Build history of the part. All positions in model axes, mm. Face numbers are marked on the shaded views. A direction names the side the tool comes from. Give positions to 0.01 mm unless a question says otherwise; leave off trailing zeros. Loops run counter-clockwise (first coordinate to the right, second up) from the corner with the lowest first, then second, coordinate; pieces in that order, holes last. Notation, with made-up numbers: (-11, 47.25) - (22, 47.25) arc R27 cw to (22, 63.25) - close; hole circle Ø3 at (72, 73). An arc over 180 degrees is marked (long way). Return JSON: item names as keys, results as strings. Group by question number.
1) Slice it at A-A (z = -26.5). List the corners of the cut face in (x, y), and give its area (3 significant figures).
2) Mould opens along Y. For the marked faces 1, 2 and 3 say: released by +Y, released by -Y, zero draft, split by the parting line, or undercut.
3) Slice it at C-C (y = 14). List the corners of the cut face in (x, z).
4) 3-axis set-ups, long thin cutter, end or side, ignore diameter. For the marked faces 4, 5, 6, 7 and 8: which of +Z, -Z, +X, -X, +Y, -Y reach the whole face in a straight line?
5) Slice it at B-B (x = 26.5). List the corners of the cut face in (y, z), and give its area (3 significant figures).
6) Slice it at D-D (z = -11). List the corners of the cut face in (x, y).
7) Drill centre lines: probe 1 along Z at (x, y) = (47.5, 4); probe 2 along X at (y, z) = (10.5, -23); probe 3 along Y at (x, z) = (44, -5). Where is each one in solid material? Low to high. Write a range as from..to.
8) Drop flat-ended pins along their axis: pin 1 (1 mm diameter, centred on x = 31, y = 4, fed in from +Z); pin 2 (5.5 mm diameter, centred on x = 10.35, y = 10.35, fed in from -Z); pin 3 (1.5 mm diameter, centred on x = 20.5, y = -16, fed in from -Z); pin 4 (5.5 mm diameter, centred on x = 9, y = 14, fed in from -Z). Give the stop position or say it passes through.
```python
from build123d import *

# Parameters (mm, degrees)
BOSS_EXTRUDE1_DEPTH  = 20.701
SKETCH2_R            = 1
CUT_EXTRUDE1_DEPTH   = 93.545558787
SKETCH3_R            = 1
CUT_EXTRUDE2_DEPTH   = 12.7
SKETCH4_R            = 1
BOSS_EXTRUDE3_DEPTH  = 5.08
SKETCH5_W            = 5.08
SKETCH5_H            = 5.08
BOSS_EXTRUDE4_DEPTH  = 5.08
SKETCH6_W            = 5.08
SKETCH6_H            = 5.08
BOSS_EXTRUDE5_DEPTH  = 5.08
SKETCH7_W            = 2.54
SKETCH7_H            = 15
CUT_EXTRUDE3_DEPTH   = 108.238791728
SKETCH8_W            = 25.4
SKETCH8_H            = 32.87751569
CUT_EXTRUDE4_DEPTH   = 99.137252123
BOSS_EXTRUDE6_DEPTH  = 5.08
BOSS_EXTRUDE9_START  = -5.08
SKETCH12_R           = 1
BOSS_EXTRUDE9_DEPTH  = 5.08
SKETCH13_R           = 1
BOSS_EXTRUDE10_DEPTH = 24.4
CUT_EXTRUDE5_DEPTH   = 30
SKETCH11_R           = 4.5
CUT_EXTRUDE6_DEPTH   = 40
SKETCH16_R           = 3.175
SKETCH16_R_2         = 4.7625
SKETCH16_R_3         = 2.5
CUT_EXTRUDE7_DEPTH   = 40


with BuildPart() as part:
    # Sketch1 → Boss-Extrude1 (new body)
    with BuildSketch(Plane(origin=(0, 0, 0), x_dir=(1, 0, 0), z_dir=(0, 1, 0))):
        Polygon((86.5505, 0), (86.5505, 25.4), (81.4705, 25.4), (81.4705, 10.16), (76.3905, 5.08), (81.4705, 5.08), (81.4705, 0), align=None)
        Polygon((20.701, 10.16), (20.701, 25.4), (0, 25.4), (0, 0), (81.4705, 0), (81.4705, 5.08), (76.3905, 5.08), (25.781, 5.08), (20.701, 5.08), align=None)
        Polygon((20.701, 10.16), (25.781, 5.08), (20.701, 5.08), align=None)
    extrude(amount=BOSS_EXTRUDE1_DEPTH)

    # Sketch2 → Cut-Extrude1 (cut, through all)
    with BuildSketch(Plane(origin=(0, 0, -25.4), x_dir=(-1, 0, 0), z_dir=(0, 0, -1))):
        with Locations((-10.3505, 10.3505)):
            Circle(SKETCH2_R)
    extrude(amount=-CUT_EXTRUDE1_DEPTH, mode=Mode.SUBTRACT)

    # Sketch3 → Cut-Extrude2 (cut)
    with BuildSketch(Plane.XY):
        with Locations((50.970999912, 10.3505)):
            Circle(SKETCH3_R)
    extrude(amount=-CUT_EXTRUDE2_DEPTH, mode=Mode.SUBTRACT)

    # Sketch4 → Boss-Extrude3 (add)
    with BuildSketch(Plane.XY):
        with BuildLine():
            Line((40.280941282, 0), (27.580941282, 0))
            Line((27.580941282, 0), (25.4, 0))
            Line((25.4, 0), (0, 0))
            Line((0, 0), (16.608872552, -28.493600659))
            ThreePointArc((16.608872552, -28.493600659), (30.893397103, -34.358409309), (40.280941282, -22.098))
            Line((40.280941282, -22.098), (40.280941282, 0))
        make_face()
        with Locations((20.138741282, -22.098)):
            Circle(SKETCH4_R, mode=Mode.SUBTRACT)
        with BuildLine():
            ThreePointArc((26.580941282, -22.098), (26.873834501, -21.390893219), (27.580941282, -21.098))
            ThreePointArc((27.580941282, -21.098), (28.288048063, -21.390893219), (28.580941282, -22.098))
            ThreePointArc((28.580941282, -22.098), (27.580941282, -23.098), (26.580941282, -22.098))
        make_face(mode=Mode.SUBTRACT)
        with BuildLine():
            ThreePointArc((36.023141282, -22.098), (35.023141282, -23.098), (34.023141282, -22.098))
            ThreePointArc((34.023141282, -22.098), (35.023141282, -21.098), (36.023141282, -22.098))
        make_face(mode=Mode.SUBTRACT)
    extrude(amount=-BOSS_EXTRUDE3_DEPTH)

    # Sketch5 → Boss-Extrude4 (add)
    with BuildSketch(Plane(origin=(0, 0, -25.4), x_dir=(-1, 0, 0), z_dir=(0, 0, -1))):
        with Locations((-2.54, 2.54)):
            Rectangle(SKETCH5_W, SKETCH5_H)
        with Locations((-2.54, 18.161)):
            Rectangle(SKETCH5_W, SKETCH5_H)
        with Locations((-18.161, 18.161)):
            Rectangle(SKETCH5_W, SKETCH5_H)
        with Locations((-18.161, 2.54)):
            Rectangle(SKETCH5_W, SKETCH5_H)
    extrude(amount=BOSS_EXTRUDE4_DEPTH)

    # Sketch6 → Boss-Extrude5 (add)
    with BuildSketch(Plane(origin=(0, 0, -25.4), x_dir=(-1, 0, 0), z_dir=(0, 0, -1))):
        with Locations((-84.0105, 18.161)):
            Rectangle(SKETCH6_W, SKETCH6_H)
        with Locations((-84.0105, 2.54)):
            Rectangle(SKETCH6_W, SKETCH6_H)
    extrude(amount=BOSS_EXTRUDE5_DEPTH)

    # Sketch7 → Cut-Extrude3 (cut, through all)
    with BuildSketch(Plane(origin=(0, 20.701, 0), x_dir=(1, 0, 0), z_dir=(0, 1, 0))):
        with Locations((82.7405, 22.98)):
            Rectangle(SKETCH7_W, SKETCH7_H)
        with Locations((19.431, 22.98)):
            Rectangle(SKETCH7_W, SKETCH7_H)
    extrude(amount=-CUT_EXTRUDE3_DEPTH, mode=Mode.SUBTRACT)

    # Sketch8 → Cut-Extrude4 (cut, through all)
    with BuildSketch(Plane(origin=(0, 0, 0), x_dir=(-1, 0, 0), z_dir=(0, -1, 0))):
        with Locations((-73.8505, 16.438757845)):
            Rectangle(SKETCH8_W, SKETCH8_H)
    extrude(amount=-CUT_EXTRUDE4_DEPTH, mode=Mode.SUBTRACT)

    # Sketch9 → Boss-Extrude6 (add)
    with BuildSketch(Plane.XY):
        with BuildLine():
            Line((8.304436276, -28.493600659), (16.608872552, -28.493600659))
            Line((16.608872552, -28.493600659), (0, 0))
            Line((0, 0), (0, -14.24680033))
            Line((0, -14.24680033), (3.648627535, -20.506258075))
            ThreePointArc((3.648627535, -20.506258075), (4.650419602, -20.503139192), (5.152218138, -21.370200495))
            ThreePointArc((5.152218138, -21.370200495), (5.01927944, -21.868401958), (4.655808741, -22.234142914))
            Line((4.655808741, -22.234142914), (8.304436276, -28.493600659))
        make_face()
        with BuildLine():
            Line((0, -28.493600659), (8.304436276, -28.493600659))
            Line((8.304436276, -28.493600659), (4.655808741, -22.234142914))
            ThreePointArc((4.655808741, -22.234142914), (3.288275718, -21.873791098), (3.648627535, -20.506258075))
            Line((3.648627535, -20.506258075), (0, -14.24680033))
            Line((0, -14.24680033), (0, -28.493600659))
        make_face()
    extrude(amount=-BOSS_EXTRUDE6_DEPTH)

    # Sketch12 → Boss-Extrude9 (add)
    with BuildSketch(Plane(origin=(0, 0, -5.08), x_dir=(-1, 0, 0), z_dir=(0, 0, -1)).offset(BOSS_EXTRUDE9_START)):
        with Locations((-4.152218138, -21.370200495)):
            Circle(SKETCH12_R)
        with Locations((-20.138741282, -22.098)):
            Circle(SKETCH12_R)
        with Locations((-27.580941282, -22.098)):
            Circle(SKETCH12_R)
        with Locations((-35.023141282, -22.098)):
            Circle(SKETCH12_R)
        with Locations((-50.970999912, 10.3505)):
            Circle(SKETCH12_R)
    extrude(amount=BOSS_EXTRUDE9_DEPTH)

    # Sketch13 → Boss-Extrude10 (add)
    with BuildSketch(Plane(origin=(0, 0, -25.4), x_dir=(-1, 0, 0), z_dir=(0, 0, -1))):
        with Locations((-10.3505, 10.3505)):
            Circle(SKETCH13_R)
    extrude(amount=-BOSS_EXTRUDE10_DEPTH)

    # Sketch15 → Cut-Extrude5 (cut)
    with BuildSketch(Plane(origin=(0, 20.701, 0), x_dir=(1, 0, 0), z_dir=(0, 1, 0))):
        Polygon((18.161, 15.48), (18.161, 12.717664049), (20.701, 10.16), (20.701, 15.48), align=None)
    extrude(amount=-CUT_EXTRUDE5_DEPTH, mode=Mode.SUBTRACT)

    # Sketch11 → Cut-Extrude6 (cut)
    with BuildSketch(Plane.XY):
        with Locations((10.3505, 10.3505)):
            Circle(SKETCH11_R)
    extrude(amount=-CUT_EXTRUDE6_DEPTH, mode=Mode.SUBTRACT)

    # Sketch16 → Cut-Extrude7 (cut)
    with BuildSketch(Plane.XY):
        with Locations((27.580941282, -22.098)):
            Circle(SKETCH16_R)
        with Locations((50.970999912, 10.3505)):
            Circle(SKETCH16_R_2)
        with Locations((4.152218138, -21.370200495)):
            Circle(SKETCH16_R_3)
    extrude(amount=-CUT_EXTRUDE7_DEPTH, mode=Mode.SUBTRACT)


solid = part.part
```
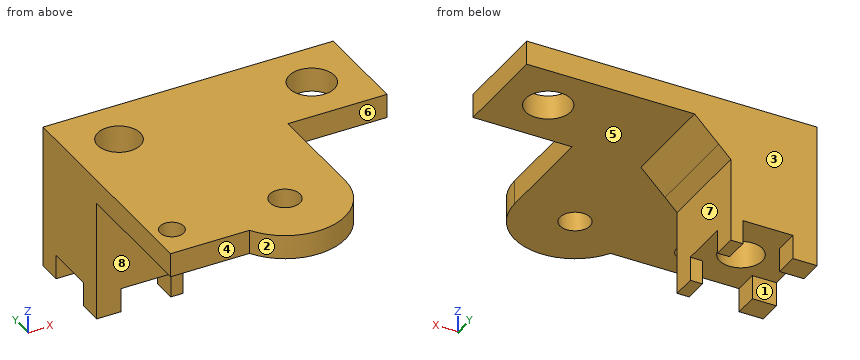
Results:
{
 "1": {"outline": "(0, 0) - (5.08, 0) - (5.08, 5.08) - (0, 5.08) - close; (0, 15.62) - (5.08, 15.62) - (5.08, 20.7) - (0, 20.7) - close; (15.62, 0) - (18.16, 0) - (18.16, 5.08) - (15.62, 5.08) - close; (15.62, 15.62) - (18.16, 15.62) - (18.16, 20.7) - (15.62, 20.7) - close", "area": "77.4 mm2"},
 "2": {"face 1": "undercut", "face 2": "released by -Y", "face 3": "released by +Y"},
 "3": {"outline": "(0, -25.4) - (7.72, -25.4) - (7.72, 0) - (0, 0) - close; (12.98, -25.4) - (18.16, -25.4) - (18.16, -12.72) - (20.7, -10.16) - (25.78, -5.08) - (47.91, -5.08) - (47.91, 0) - (12.98, 0) - close; (54.03, -5.08) - (61.15, -5.08) - (61.15, 0) - (54.03, 0) - close"},
 "4": {"face 4": "+Z, -Z, -X, -Y", "face 5": "-Z, +X, -Y", "face 6": "+Z, -Z, +X, -Y", "face 7": "-Z, +X, +Y, -Y", "face 8": "-Z, +X, -X, -Y"},
 "5": {"outline": "(-34.75, -5.08) - (-25.08, -5.08) - (-25.08, 0) - (-34.75, 0) - close; (-19.11, -5.08) - (20.7, -5.08) - (20.7, 0) - (-19.11, 0) - close", "area": "251 mm2"},
 "6": {"outline": "(0, 0) - (19.87, 0) - (19.87, 20.7) - (0, 20.7) - close; hole circle Ø9 at (10.35, 10.35)"},
 "7": {"probe 1": "-5.08..0", "probe 2": "0..5.85, 14.85..18.16", "probe 3": "0..20.7"},
 "8": {"pin 1": "z = 0", "pin 2": "through", "pin 3": "z = -5.08", "pin 4": "z = -25.4"}
}
